Read the model definition and answer for the solid it produces. Units are mm, in the model's axes. A direction names the side the tool comes from. Coordinates: 2 decimals unless noted, no trailing zeros. Order: outer loops, then holes, each group sorted by start corner. A loop starts at its lowest first (then second) coordinate and runs counter-clockwise, first axis right, second up. Notation, with made-up numbers: M 19,56.25 L 34,56.25 A17 ccw 34,63.25 Z; hole C 63,-13.5 d2. An arc over 180 degrees is marked long. Put each result on its own line as item: value.
from build123d import *

# Parameters (mm, degrees)
F0_W             = 31.75
F0_H             = 63.5
F0_W_2           = 7.62
F0_H_2           = 10.8501603827
F1_DEPTH         = 1.6
F2_W             = 6.985
F2_H             = 1.6
F3_DEPTH         = 6.35
F5_DEPTH         = 25.4
F5_COPIES2_COUNT = 2
F5_COPIES2_PITCH = 70.023265


# Not quite as in the source:
# - a feature of the source that left no trace in its solid (it failed there, or was rolled back) is left out
# - a pattern or mirror of a feature is missing from the dataset's text; its kind, count and spacing are read off the source's solid
# - a feature names something its author has since deleted; it is built from what else it names


with BuildPart() as f1:
    # F0 (on Top) → F1 (new body)
    with BuildSketch(Plane.XY):
        with Locations((15.875, 31.75)):
            Rectangle(F0_W, F0_H)
        with Locations((15.875, 20.8916743286)):
            Rectangle(F0_W_2, F0_H_2, mode=Mode.SUBTRACT)
    extrude(amount=F1_DEPTH)

    # F2 (on face) → F3 (join)
    with BuildSketch(Plane.XZ):
        with Locations((3.4925, 0.8)):
            Rectangle(F2_W, F2_H)
        with Locations((28.2575, 0.8)):
            Rectangle(F2_W, F2_H)
    extrude(amount=F3_DEPTH)

    # F4 (on face) → F5 (cut)
    with BuildSketch(Plane.XY.offset(1.6)):
        with BuildLine():
            ThreePointArc((5.29375, -4.35), (3.0318335149, -3.4130835149), (3.96875, -5.675))
            Line((3.96875, -5.675), (3.96875, -4.35))
            Line((3.96875, -4.35), (5.29375, -4.35))
        make_face()
        with BuildLine():
            Line((3.96875, -4.35), (3.96875, -5.675))
            ThreePointArc((3.96875, -5.675), (4.9056664851, -5.2869164851), (5.29375, -4.35))
            Line((5.29375, -4.35), (3.96875, -4.35))
        make_face()
    f5 = extrude(amount=-F5_DEPTH, mode=Mode.SUBTRACT)

    # F5_copies: F5 across plane
    add(f5.mirror(Plane.ZX.offset(28.575)), mode=Mode.SUBTRACT)

    # F5_copies1: F5 across plane
    add(f5.mirror(Plane(origin=(15.875, 0, 0), x_dir=(0, 0, 1), z_dir=(1, 0, 0))), mode=Mode.SUBTRACT)

    # F5_copies2: F5 ×2
    with Locations(*[Vector(0.3400655477, 0.940401735, 0) * (i * F5_COPIES2_PITCH) for i in range(1, F5_COPIES2_COUNT)]):
        add(f5, mode=Mode.SUBTRACT)


solid = f1.part
Q1. Given pin 1 (2 mm diameter, centred on x = 3.97, y = 61.5, fed in from +Z); pin 2 (0.5 mm diameter, centred on x = 16, z = 0.5, fed in from -Y), each flat-ended and moving along its own axis, determine where each tip first touches the part or whether it passes through.
Answers below:
pin 1: passes through
pin 2: stops at y = 0
Q2. Find section C-C on x = 22.5. Write down the section's boundary in (y, z), plus the area to 3 significant figures.
Answers below:
outline: M 0,0 L 63.5,0 L 63.5,1.6 L 0,1.6 Z
area: 102 mm^2
Q3. Consider line 1 along Y through (x, z) = (4, 1.1); line 2 along X through (y, z) = (-4.35, 0.55) (3 decimals); line 3 along X through (y, z) = (61.5, 1.2). Determine where each line is inside the solid, lowest interval first.
Answers below:
line 1: y = -6.35 to -5.67, -3.03 to 60.18, 62.82 to 63.5
line 2: x = 0 to 2.644, 5.294 to 6.985, 24.765 to 26.456, 29.106 to 31.75
line 3: x = 0 to 2.64, 5.29 to 26.46, 29.11 to 31.75
Q4. A tool of negligible diameter and unlimited length cuts with its end or side. For faces 1 (the face through (16, 0, 1)), 2 (the face through (16, 29, 0)), 3 (the face through (12.065, 21, 1)), from which of +Z, -Z, +X, -X, +Y, -Y can it reach the whole face along a straight path? Write none if from no direction.
Answers below:
face 1: +Z, -Z, -Y
face 2: -Z, +X, -X, +Y, -Y
face 3: +Z, -Z
Q5. Find section A-A on y = 24. Write down the section's boundary in (x, z) (3 decimals), plus the area to 3 significant figures.
Answers below:
outline: M 0,0 L 12.065,0 L 12.065,1.6 L 0,1.6 Z; M 19.685,0 L 31.75,0 L 31.75,1.6 L 19.685,1.6 Z
area: 38.6 mm^2
Q6. For a pull along X with two mould halves and no side action, classify faces 4 (the face through (19.685, 21, 1)), 5 (the face through (16, 26.317, 1)), 6 (the face through (28, -6.35, 1)), 7 (the face through (0, 29, 1)) as +X half, -X half, draft (parallel to the pull), parting line (faces both ways), or undercut.
Answers below:
face 4: undercut
face 5: undercut
face 6: draft
face 7: -X half
Q7. Find section B-B on z = 0.95. Write down the section's boundary in (x, y) (3 decimals), plus the area to 3 significant figures.
Answers below:
outline: M 0,-6.35 L 6.985,-6.35 L 6.985,0 L 24.765,0 L 24.765,-6.35 L 31.75,-6.35 L 31.75,63.5 L 0,63.5 Z; hole C 3.969,-4.35 d2.65; hole C 3.969,61.5 d2.65; hole M 12.065,15.467 L 19.685,15.467 L 19.685,26.317 L 12.065,26.317 Z; hole C 27.781,-4.35 d2.65; hole C 27.781,61.5 d2.65
area: 2,000 mm^2
